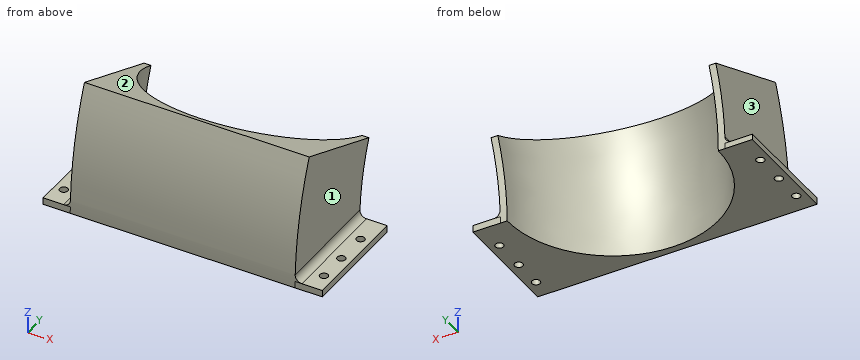
```python
from build123d import *

# Parameters (mm, degrees)
REVOLVE8_ANGLE         = 22.5
BOSS_EXTRUDE3_START    = 12.7
BOSS_EXTRUDE3_DEPTH    = 12.7
BOSS_EXTRUDE4_DEPTH    = 12.7
SKETCH12_R             = 1.905
CUT_EXTRUDE4_DEPTH     = 3.175
SKETCH13_R             = 1.905
CUT_EXTRUDE5_DEPTH     = 3.175
FLANGE_REINFORCEMENT_R = 3.175


with BuildPart() as part:
    # Sketch9 → Revolve8 (revolve)
    with BuildSketch(Plane.XY):
        with BuildLine():
            Line((-49.2252, -98.425), (-52.4002, -98.425))
            Line((-52.4002, -98.425), (-52.4002, -150.8252))
            Line((-52.4002, -150.8252), (52.4002, -150.8252))
            Line((52.4002, -150.8252), (52.4002, -98.425))
            Line((52.4002, -98.425), (49.2252, -98.425))
            ThreePointArc((49.2252, -98.425), (0, -147.6502), (-49.2252, -98.425))
        make_face()
    revolve(axis=Axis((-38.048924234, 0, 0), (-1, 0, 0)), revolution_arc=REVOLVE8_ANGLE)

    # Sketch11 → Boss-Extrude3 (add)
    with BuildSketch(Plane.ZY.offset(52.4002).offset(BOSS_EXTRUDE3_START)):
        with BuildLine():
            Line((0, -98.425), (0, -150.8252))
            ThreePointArc((0, -150.8252), (1.5875, -150.816845209), (3.174824124, -150.791781762))
            Line((3.174824124, -150.791781762), (2.623242695, -98.390036197))
            ThreePointArc((2.623242695, -98.390036197), (1.311737846, -98.416258661), (0, -98.425))
        make_face()
    extrude(amount=-BOSS_EXTRUDE3_DEPTH)

    # Sketch10 → Boss-Extrude4 (add)
    with BuildSketch(Plane(origin=(52.4002, 0, 0), x_dir=(0, 0, -1), z_dir=(1, 0, 0))):
        with BuildLine():
            Line((0, -98.425), (0, -150.8252))
            Line((0, -150.8252), (-3.174824124, -150.791781762))
            Line((-3.174824124, -150.791781762), (-3.174824124, -98.37378267))
            ThreePointArc((-3.174824124, -98.37378267), (-1.587618613, -98.412194834), (0, -98.425))
        make_face()
    extrude(amount=BOSS_EXTRUDE4_DEPTH)

    # Sketch12 → Cut-Extrude4 (cut)
    with BuildSketch(Plane.XY.offset(3.174824124)):
        with Locations((60.550186424, -111.886000657)):
            Circle(SKETCH12_R)
        with Locations((60.550186424, -141.566764633)):
            Circle(SKETCH12_R)
        with Locations((60.550186424, -127.4445)):
            Circle(SKETCH12_R)
    extrude(amount=-CUT_EXTRUDE4_DEPTH, mode=Mode.SUBTRACT)

    # Sketch13 → Cut-Extrude5 (cut)
    with BuildSketch(Plane(origin=(0, -0.008353865, 1.587675876), x_dir=(1, 0, 0), z_dir=(-8.55203915581382e-15, 0.010525429437517081, 0.9999446061333377))):
        with Locations(Location((-60.754019077, -141.521938379, 0), (0, 0, 270))):
            Circle(SKETCH13_R)
        with Locations(Location((-60.754019077, -112.479497113, 0), (0, 0, 270))):
            Circle(SKETCH13_R)
        with Locations(Location((-60.754019077, -127.4445, 0), (0, 0, 270))):
            Circle(SKETCH13_R)
    extrude(amount=-CUT_EXTRUDE5_DEPTH, mode=Mode.SUBTRACT)

    # Flange Reinforcement
    # the kernel refuses this fillet: 3.175 mm, written as the material it adds along each edge
    with BuildSketch(Plane(origin=(-52.4002, -158.728842073, 3.258369721), x_dir=(-8.951719505639043e-15, 0.010525429437517086, 0.9999446061333377), z_dir=(-8.181600859283099e-15, 0.9999446061333378, -0.01052542943751709))) as flange_reinforcement_piece_1_section:
        with BuildLine():
            CenterArc((FLANGE_REINFORCEMENT_R, -FLANGE_REINFORCEMENT_R), FLANGE_REINFORCEMENT_R, 90, 90)
            Line((0, -FLANGE_REINFORCEMENT_R), (0, 0))
            Line((0, 0), (FLANGE_REINFORCEMENT_R, 0))
        make_face()
    flange_reinforcement_piece_1 = extrude(amount=68.279648461, mode=Mode.PRIVATE)
    flange_reinforcement_piece_1 = flange_reinforcement_piece_1 - Plane(origin=(-53.118961538, 0, 0), x_dir=(0, -1, 0), z_dir=(-1, 0, 0)) * Cylinder(98.425, 150, mode=Mode.PRIVATE)
    flange_reinforcement_piece_1 = flange_reinforcement_piece_1 & Plane(origin=(-53.118961538, 0, 0), x_dir=(0, -1, 0), z_dir=(1, 0, 0)) * Cylinder(150.8252, 150, mode=Mode.PRIVATE)
    add(flange_reinforcement_piece_1)
    with BuildSketch(Plane(origin=(52.4002, -158.729281762, 3.174824124), x_dir=(0, 0, 1), z_dir=(0, 1, 0))) as flange_reinforcement_piece_2_section:
        with BuildLine():
            CenterArc((FLANGE_REINFORCEMENT_R, FLANGE_REINFORCEMENT_R), FLANGE_REINFORCEMENT_R, 180, 90)
            Line((0, FLANGE_REINFORCEMENT_R), (0, 0))
            Line((0, 0), (FLANGE_REINFORCEMENT_R, 0))
        make_face()
    flange_reinforcement_piece_2 = extrude(amount=68.292999092, mode=Mode.PRIVATE)
    flange_reinforcement_piece_2 = flange_reinforcement_piece_2 - Plane(origin=(53.118931151, 0, 0), x_dir=(0, -1, 0), z_dir=(-1, 0, 0)) * Cylinder(98.425, 150, mode=Mode.PRIVATE)
    flange_reinforcement_piece_2 = flange_reinforcement_piece_2 & Plane(origin=(53.118931151, 0, 0), x_dir=(0, -1, 0), z_dir=(1, 0, 0)) * Cylinder(150.8252, 150, mode=Mode.PRIVATE)
    add(flange_reinforcement_piece_2)


solid = part.part
```
The model under review builds one solid part; all positions refer to its coordinate system, in mm. Face numbers are marked on the shaded views. A direction names the side the tool comes from. Round coordinates to 2 decimals unless told otherwise and drop trailing zeros. Order: outer loops, then holes, each group sorted by start corner. A loop starts at its lowest first (then second) coordinate and runs counter-clockwise, first axis right, second up. Notation, with made-up numbers: (9.5, -24.75) -> (40.5, -24.75) arc R38 ccw to (40.5, 14.25) -> close; hole circle Ø2 at (-12.75, -10.5). An arc over 180 degrees is marked (long way). One line per item, written item: value. Start each with the question number.
Q1. Clearance check with flat-ended pins moving along their axes: pin 1 Ø4.5 at (x, y) = (60.55, -141.57) entering from +Z; pin 2 Ø2 at (x, z) = (-48, 34) entering from -Y; pin 3 Ø8 at (y, z) = (-130, 8.5) entering from +X. State where each tip first meets the part, or that it passes through.
Q2. Take a section at C-C (x = 34). Write out the cut boundary in (y, z), and give its area (3 significant figures).
Q3. Machinability: for the marked faces 1, 2 and 3, which of the approach directions +Z, -Z, +X, -X, +Y, -Y give a long, thin tool a straight path to every point of the face, cutting with its end or side? Answer none if there is none.
Q4. Take a section at B-B (x = -32). Write out the cut boundary in (y, z).
Q5. Wall thickness on line 1 (X direction, y = -97, z = 24.5); line 2 (X direction, y = -114, z = 2.5); line 3 (X direction, y = -107.5, z = 3): over which ranges is each line inside the solid? List them lowest first.
Q6. Take a section at A-A (x = 54). Write out the cut boundary in (y, z) (3 decimals), and give its area (3 significant figures).
Reported:
1. pin 1: stops at z = 3.17
1. pin 2: stops at y = -147.17
1. pin 3: stops at x = 52.99
2. outline: (-150.83, 0) -> (-134.02, 0) arc R134.02 cw to (-123.82, 51.29) -> (-139.34, 57.72) arc R150.83 ccw to start
2. area: 940 mm2
3. face 1: +Z, +X, +Y, -Y
3. face 2: +Z, +X, -X, +Y
3. face 3: +Z, -X, +Y, -Y
4. outline: (-150.83, 0) -> (-135.83, 0) arc R135.83 cw to (-125.49, 51.98) -> (-139.34, 57.72) arc R150.83 ccw to start
5. line 1: x = -52.4 to -49.2, 49.2 to 52.4
5. line 2: x = -65.1 to -61.91, -59.6 to -46.69, 46.69 to 65.1
5. line 3: x = -54.27 to -48.37, 48.37 to 65.1
6. outline: (-150.825, 0) -> (-98.425, 0) arc R98.425 cw to (-98.374, 3.175) arc R98.425 cw to (-98.359, 3.593) -> (-150.782, 3.593) arc R150.825 ccw to (-150.792, 3.175) -> close
6. area: 188 mm2
